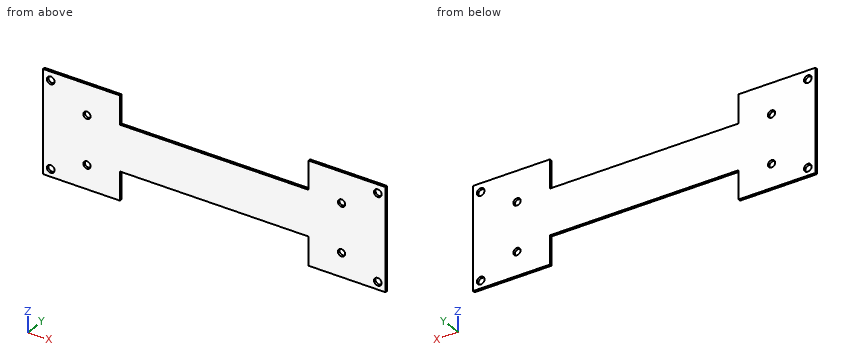
```python
from build123d import *

# Parameters (mm, degrees)
SKETCH1_W          = 178
SKETCH1_H          = 54
BASE_FLANGE1_DEPTH = 1.2
SKETCH2_R          = 1.9
CUT_EXTRUDE1_DEPTH = 10
SKETCH3_W          = 98
SKETCH3_H          = 15
CUT_EXTRUDE2_DEPTH = 10
SKETCH4_R          = 2
CUT_EXTRUDE3_DEPTH = 10
SKETCH5_R          = 2
CUT_EXTRUDE4_DEPTH = 10


# Sheet-metal steps are written as plain solids
with BuildPart() as part:
    # Sketch1 → Base-Flange1 (new body)
    with BuildSketch(Plane(origin=(0, 0, 0), x_dir=(1, 0, 0), z_dir=(0, 1, 0))):
        with Locations((25.098152401, 5.183748797)):
            Rectangle(SKETCH1_W, SKETCH1_H)
    extrude(amount=-BASE_FLANGE1_DEPTH)

    # Sketch2 → Cut-Extrude1 (cut)
    with BuildSketch(Plane(origin=(0, 0, 0), x_dir=(1, 0, 0), z_dir=(0, 1, 0))):
        with Locations(Location((91.253152401, -5.816251203, 0), (0, 0, 270))):
            Circle(SKETCH2_R)
        with Locations(Location((-41.056847599, -5.816251203, 0), (0, 0, 270))):
            Circle(SKETCH2_R)
        with Locations(Location((91.253152401, 19.713748797, 0), (0, 0, 270))):
            Circle(SKETCH2_R)
        with Locations(Location((-41.056847599, 19.713748797, 0), (0, 0, 270))):
            Circle(SKETCH2_R)
    extrude(amount=-CUT_EXTRUDE1_DEPTH, mode=Mode.SUBTRACT)

    # Sketch3 → Cut-Extrude2 (cut)
    with BuildSketch(Plane(origin=(0, 0, 0), x_dir=(1, 0, 0), z_dir=(0, 1, 0))):
        with Locations((25.098152401, -14.316251203)):
            Rectangle(SKETCH3_W, SKETCH3_H)
        with Locations((25.098152401, 24.683748797)):
            Rectangle(SKETCH3_W, SKETCH3_H)
    extrude(amount=-CUT_EXTRUDE2_DEPTH, mode=Mode.SUBTRACT)

    # Sketch4 → Cut-Extrude3 (cut)
    with BuildSketch(Plane(origin=(0, 0, 0), x_dir=(1, 0, 0), z_dir=(0, 1, 0))):
        with Locations(Location((110.098152401, -17.316251203, 0), (0, 0, 270))):
            Circle(SKETCH4_R)
        with Locations(Location((110.098152401, 28.183748797, 0), (0, 0, 270))):
            Circle(SKETCH4_R)
    extrude(amount=-CUT_EXTRUDE3_DEPTH, mode=Mode.SUBTRACT)

    # Sketch5 → Cut-Extrude4 (cut)
    with BuildSketch(Plane(origin=(0, 0, 0), x_dir=(1, 0, 0), z_dir=(0, 1, 0))):
        with Locations(Location((-59.901847599, -17.316251203, 0), (0, 0, 270))):
            Circle(SKETCH5_R)
        with Locations(Location((-59.901847599, 28.183748797, 0), (0, 0, 270))):
            Circle(SKETCH5_R)
    extrude(amount=-CUT_EXTRUDE4_DEPTH, mode=Mode.SUBTRACT)


solid = part.part
```
Input: part model. Units: mm. Frame: model coordinates. Round coordinates to 2 decimals unless told otherwise and drop trailing zeros. Loops run counter-clockwise (first coordinate to the right, second up) from the corner with the lowest first, then second, coordinate; pieces in that order, holes last. Notation, with made-up numbers: (-25, -1) - (28, -1) arc R32 cw to (28, 31) - close; hole circle Ø2 at (47.25, 55). An arc over 180 degrees is marked (long way). One line per item, written item: value. Start each with the question number.
(1) Section A-A, the plane z = -23.5. Return loops of the section in (x, y).
(2) Section C-C, the plane x = 60. Return loops of the section in (y, z), plus the area to 3 significant figures.
(3) Ray query, line 1 (X direction, y = -0.55, z = 6); line 2 (X direction, y = -0.2, z = 12); line 3 (X direction, y = -0.7, z = 18). Return the intervals inside material, ascending. Write a range as [from, to].
(4) Contact query for a flat-ended pin moving along its axis: P1, Ø0.6, axis at x = 43.5, y = -0.5, coming from the -Z side. Output: stop coordinate, or through.
(5) Section B-B, the plane y = -0.6. Count the separate pieces of the cut face and the enclosed holes in it, plus the area to 3 significant figures.
Results below:
1. outline: (-63.9, -1.2) - (-23.9, -1.2) - (-23.9, 0) - (-63.9, 0) - close; (74.1, -1.2) - (114.1, -1.2) - (114.1, 0) - (74.1, 0) - close
2. outline: (-1.2, -17.18) - (0, -17.18) - (0, 6.82) - (-1.2, 6.82) - close
2. area: 28.8 mm^2
3. line 1: [-63.9, -42.95], [-39.17, 89.36], [93.14, 114.1]
3. line 2: [-63.9, -23.9], [74.1, 114.1]
3. line 3: [-63.9, -61.78], [-58.02, -23.9], [74.1, 108.22], [111.98, 114.1]
4. P1: z = -17.18
5. separate pieces: 1
5. enclosed holes: 8
5. area: 6,580 mm^2
